Check sheet for the modelled part. Datum: model origin and axes. Units: mm. Face numbers are marked on the shaded views. A direction names the side the tool comes from. Coordinates: 2 decimals unless noted, no trailing zeros. Loops run counter-clockwise (first coordinate to the right, second up) from the corner with the lowest first, then second, coordinate; pieces in that order, holes last. Notation, with made-up numbers: M 72.5,-20 L 123.5,-20 A25 cw 123.5,3 Z; hole C 41.25,8 d10. An arc over 180 degrees is marked long. Write each question's results on one line, items separated by ' | '. Start each with the question number.
Autodesk Inventor part; units mm, degrees
ref_plane "YZ Plane" through (0, 0, 0) normal (1, 0, 0) x (0, 1, 0)
ref_plane "XZ Plane" through (0, 0, 0) normal (0, 1, 0) x (-1, 0, 0)
ref_plane "XY Plane" through (0, 0, 0) normal (0, 0, 1) x (1, 0, 0)
sketch "Эскиз1" plane through (0, 0, 0) normal (0, 1, 0) x (-1, 0, 0)
  circle A0 centre (0, 0) radius 5.45
  circle A1 centre (0, 0) radius 6.45
  line L0 (0, 0) -> (5.147, 3.8873)
  line L1 (0, 0) -> (5.147, -3.8873)
  point P0 (4.349, -3.2846)
  point P1 (4.349, 3.2846)
  dimension "d0" = 10.9
  dimension "d1" = 12.9
extrude "Выдавливание1" add sketch "Эскиз1" along normal blind 30 contours A0 L1 A1 L0 picked at (4.1928, 4.3939)
sketch "Эскиз2" plane through (0, 30, 0) normal (0, 1, 0) x (1, 0, 0)
  arc A0 (-4.349, -3.2846) -> (-5.2417, -2.7547) centre (-7.0503, -6.8185) ccw
  arc A1 (-5.2417, -2.7547) -> (-6.3986, -4.5605) centre (-5.676, -3.75) ccw
  line L0 (-6.3986, -4.5605) -> (-5.7273, -3.706)
  arc A2 (-5.1484, -3.8728) -> (-5.7273, -3.706) centre (-5.5167, -4.0632) ccw
  line L1 (-4.349, -3.2846) -> (-5.147, -3.8873)
  line L2 (-5.147, -3.8873) -> (-4.349, -3.2846)
  line L3 (-5.147, -3.8873) -> (-5.1484, -3.8728)
  line L4 (-0.0151, 0) -> (-3.489, 0)
  arc A3 (-5.2417, 2.7547) -> (-4.349, 3.2846) centre (-7.0503, 6.8185) ccw
  arc A4 (-5.7273, 3.706) -> (-5.1484, 3.8728) centre (-5.5167, 4.0632) ccw
  line L5 (-4.349, 3.2846) -> (-5.147, 3.8873)
  line L6 (-5.147, 3.8873) -> (-4.349, 3.2846)
  line L7 (-5.147, 3.8873) -> (-5.1484, 3.8728)
  arc A5 (-6.3986, 4.5605) -> (-5.2417, 2.7547) centre (-5.676, 3.75) ccw
  line L8 (-6.3986, 4.5605) -> (-5.7273, 3.706)
  point P0 (-5.3694, -4.0591)
  point P1 (-5.147, 3.8873)
  point P2 (-5.3694, 4.0591)
  point P3 (-5.147, 3.8873)
  dimension "d25" = 1.0859
sketch "Эскиз3" plane through (0, 30, 0) normal (0, 1, 0) x (1, 0, 0)
  arc A0 (-5.147, -3.8873) -> (-5.147, 3.8873) centre (0, 0) ccw
  line L0 (11.5, -6.95) -> (11.5, 6.95)
  arc A1 (-4.349, -3.2846) -> (-4.349, 3.2846) centre (0, 0) ccw
  line L1 (0, -6.45) -> (0, -5.45)
  line L2 (0, 5.45) -> (0, 6.45)
  line L3 (11.5, 6.95) -> (11.5, 10.95)
  line L4 (11.5, -6.95) -> (11.5, -10.95)
  line L5 (0, 1.95) -> (0, 6.45)
  line L6 (11.5, -10.95) -> (0, -10.95)
  line L7 (0, -10.95) -> (0, -6.45)
  line L8 (11.5, 10.95) -> (0, 10.95)
  line L9 (0, 10.95) -> (0, 6.45)
  arc A2 (0, -5.45) -> (0, 5.45) centre (0, 0) ccw
  dimension "d13" = 4
  dimension "d14" = 4
  dimension "d22" = 21.9
  dimension "d23" = 5.5
extrude "Выдавливание3" add sketch "Эскиз3" against normal blind 30
ref_plane "РабПлоскость1" through (11.5, 20, 4.95) normal (1, 0, 0) x (0, 0, -1)
sketch "Эскиз4" plane through (11.5, 20, 4.95) normal (1, 0, 0) x (0, 0, -1)
  line L0 (4.95, -20) -> (4.95, 10)
  line L1 (1, 10) -> (8.9, 10)
  circle A0 centre (4.95, -12) radius 5
  line L2 (14.4, -20) -> (-4.5, -20)
  circle A1 centre (4.95, 2) radius 5
  line L3 (-4.5, 10) -> (14.4, 10)
  point P0 (7.3306, 10)
  point P1 (2.5694, 10)
  point P2 (4.95, 10)
  dimension "d15" = 10
  dimension "d16" = 8
  dimension "d17" = 10
  dimension "d18" = 8
extrude "Выдавливание4" cut sketch "Эскиз4" against normal blind 2
extrude "Выдавливание5" add sketch "Эскиз2" against normal blind 30
sketch "Эскиз5" plane through (0, 30, 0) normal (0, 1, 0) x (1, 0, 0)
  arc A0 (0, 6.45) -> (-5.147, 3.8873) centre (0, 0) ccw
  line L0 (-5.147, 3.8873) -> (-5.1484, 3.8728)
  arc A1 (-5.7273, 3.706) -> (-5.1484, 3.8728) centre (-5.5167, 4.0632) ccw
  line L1 (-5.7273, 3.706) -> (-6.3986, 4.5605)
  arc A2 (-6.3986, 4.5605) -> (-5.2417, 2.7547) centre (-5.676, 3.75) ccw
  arc A3 (-5.2417, 2.7547) -> (-4.349, 3.2846) centre (-7.0503, 6.8185) ccw
  arc A4 (-4.349, -3.2846) -> (-4.349, 3.2846) centre (0, 0) ccw
  arc A5 (-4.349, -3.2846) -> (-5.2417, -2.7547) centre (-7.0503, -6.8185) ccw
  arc A6 (-5.2417, -2.7547) -> (-6.3986, -4.5605) centre (-5.676, -3.75) ccw
  line L2 (-6.3986, -4.5605) -> (-5.7273, -3.706)
  arc A7 (-5.1484, -3.8728) -> (-5.7273, -3.706) centre (-5.5167, -4.0632) ccw
  line L3 (-5.1484, -3.8728) -> (-5.147, -3.8873)
  arc A8 (-5.147, -3.8873) -> (0, -6.45) centre (0, 0) ccw
  line L4 (0, -6.45) -> (0, -10.95)
  line L5 (0, -10.95) -> (11.5, -10.95)
  line L6 (11.5, -10.95) -> (11.5, 10.95)
  line L7 (11.5, 10.95) -> (0, 10.95)
  line L8 (0, 10.95) -> (0, 6.45)
  line L9 (0, 5.45) -> (0, 6.45)
  line L10 (0, -5.45) -> (0, -6.45)
extrude "Выдавливание6" [suppressed]
sketch "Эскиз6" plane through (11.5, 30, 10.95) normal (1, 0, 0) x (0, 0, -1)
  arc A0 (15.95, -22) -> (15.95, -22) centre (10.95, -22) ccw
  arc A1 (15.95, -8) -> (15.95, -8) centre (10.95, -8) ccw
  point P0 (10.95, -30)
extrude "Выдавливание7" [suppressed]
properties part number "крепление маркера 11мм"
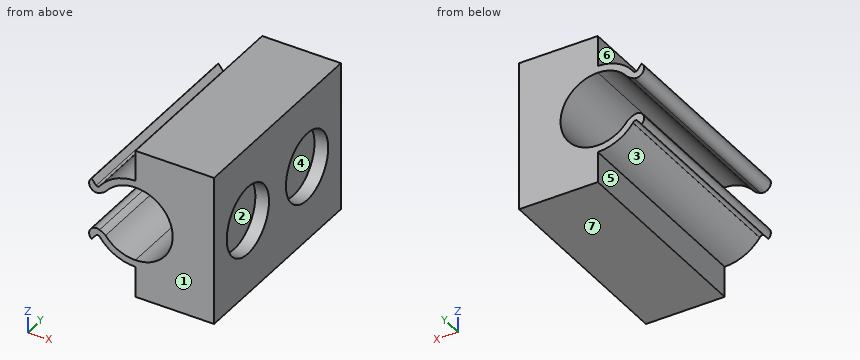
1) Section check D-D (x = 1.5). Enter the section's corners in (y, z), then the cut area to 3 significant figures.
2) Thickness scan on probe 1 along Y at (x, z) = (10.1, 0); probe 2 along Z at (x, y) = (10.8, 8); probe 3 along X at (y, z) = (6.75, 3.75). Record the ranges inside material, lowest first.
3) Set-up check for the marked faces 5, 6 and 7: record each of +Z, -Z, +X, -X, +Y, -Y from which the full face is reachable in a straight line by a thin tool's end or side.
4) Section check A-A (x = -4). Enter the section's corners in (y, z).
5) Section check B-B (z = 0). Enter the section's corners in (x, y).
6) Gauge pin test, flat ends, axial feed: P1, Ø3, axis at y = 6, z = 1.5, coming from the +X side; P2, Ø5, axis at y = 20, z = 8, coming from the -X side; P3, Ø3.5, axis at y = 19.5, z = -8.5, coming from the -X side. Record the tip position at first contact, or that the pin passes through.
7) Release check for a two-part mould opening along Z. For the marked faces 1, 2, 3 and 4 record: +Z half, -Z half, draft (parallel to the pull), parting line (faces both ways), or undercut.
Return value:
1) outline: M 0,-10.95 L 30,-10.95 L 30,-5.24 L 0,-5.24 Z; M 0,5.24 L 30,5.24 L 30,10.95 L 0,10.95 Z | area: 343 mm2
2) probe 1: y = 0 to 3, 13 to 17, 27 to 30 | probe 2: z = -10.95 to -5, 5 to 10.95 | probe 3: x = -6.76 to -5.76, -5.25 to -3.95, 3.95 to 9.5
3) face 5: -Z, -X, +Y, -Y | face 6: +Z, -X, +Y, -Y | face 7: -Z, +X, -X, +Y, -Y
4) outline: M 0,-5.06 L 30,-5.06 L 30,-3.7 L 0,-3.7 Z; M 0,3.7 L 30,3.7 L 30,5.06 L 0,5.06 Z
5) outline: M 5.45,0 L 11.5,0 L 11.5,3 L 9.5,3 L 9.5,13 L 11.5,13 L 11.5,17 L 9.5,17 L 9.5,27 L 11.5,27 L 11.5,30 L 5.45,30 Z
6) P1: stops at x = 9.5 | P2: stops at x = -3.37 | P3: stops at x = 0
7) face 1: draft | face 2: undercut | face 3: -Z half | face 4: undercut
